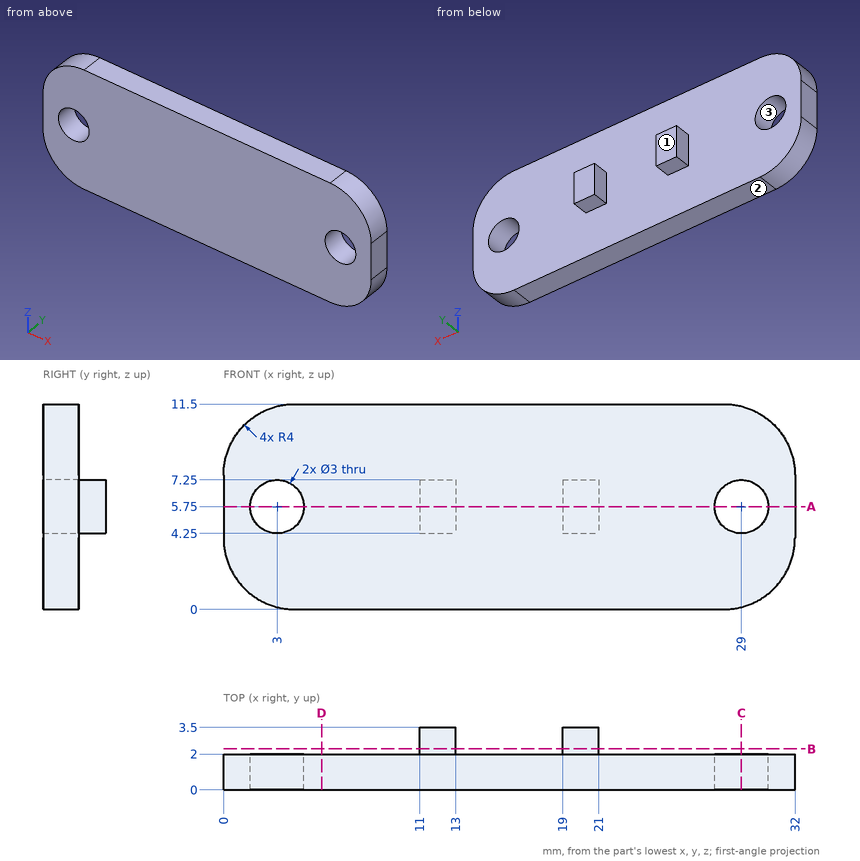
Source: three-view drawing plus pictorial views. Frame: mm from the lowest corner of the part. Give positions to 0.01 mm unless a question says otherwise; leave off trailing zeros. Write each loop counter-clockwise with the first axis right and the second up, starting at its lowest first coordinate (ties: lowest second). Pieces come first, ordered by that corner, then holes. Notation, with made-up numbers: (-15.5, 24.25) - (20.5, 24.25) arc R32 cw to (20.5, 63.25) - close; hole circle Ø7 at (12, 15). An arc over 180 degrees is marked (long way). Write item = value, one per line. Start each with the question number.
1. Section query A-A, the plane z = 5.75. Output: boundary loops of the cut face in (x, y).
2. Mould query, pull axis Z, two halves, no side actions, for the marked faces 1, 2 and 3. Classes: released by +Z, released by -Z, zero draft, split by the parting line, or undercut.
3. Ray query, L1, parallel to X at y = 0.55, z = 5.75; L2, parallel to X at y = 2.4, z = 6; L3, parallel to Z at x = 2, y = 1.5. Return the intervals inside material, ascending.
4. Section query C-C, the plane x = 29. Output: boundary loops of the cut face in (y, z).
5. Section query B-B, the plane y = 2.3. Output: boundary loops of the cut face in (x, z).
6. Section query D-D, the plane x = 5.5. Output: boundary loops of the cut face in (y, z), then the cut area to 3 significant figures.
7. First-contact query: pin 1 Ø0.8 at (x, y) = (12, 3) entering from +Z; pin 2 Ø0.8 at (y, z) = (3, 6) entering from -X; pin 3 Ø3 at (x, z) = (10.5, 1.5) entering from +Y. Flat tips, straight axial feed; report the tip coordinate or a pass-through.
Check sheet entries:
q1.outline = (0, 0) - (1.5, 0) - (1.5, 2) - (0, 2) - close; (4.5, 0) - (27.5, 0) - (27.5, 2) - (21, 2) - (21, 3.5) - (19, 3.5) - (19, 2) - (13, 2) - (13, 3.5) - (11, 3.5) - (11, 2) - (4.5, 2) - close; (30.5, 0) - (32, 0) - (32, 2) - (30.5, 2) - close
q2.face_1 = zero draft
q2.face_2 = released by -Z
q2.face_3 = undercut
q3.L1 = 0 to 1.5, 4.5 to 27.5, 30.5 to 32
q3.L2 = 11 to 13, 19 to 21
q3.L3 = 0.54 to 4.63, 6.87 to 10.96
q4.outline = (0, 0.13) - (2, 0.13) - (2, 4.25) - (0, 4.25) - close; (0, 7.25) - (2, 7.25) - (2, 11.37) - (0, 11.37) - close
q5.outline = (11, 4.25) - (13, 4.25) - (13, 7.25) - (11, 7.25) - close; (19, 4.25) - (21, 4.25) - (21, 7.25) - (19, 7.25) - close
q6.outline = (0, 0) - (2, 0) - (2, 11.5) - (0, 11.5) - close
q6.area = 23.0 mm2
q7.pin_1 = 7.25
q7.pin_2 = 11
q7.pin_3 = 2
